Geometry: final body of the model. Coordinates: model frame, mm. Give positions to 0.01 mm unless a question says otherwise; leave off trailing zeros. Order: outer loops, then holes, each group sorted by start corner. A loop starts at its lowest first (then second) coordinate and runs counter-clockwise, first axis right, second up. Notation, with made-up numbers: (84, -22) - (139, -22) arc R31 ccw to (139, 17) - close; hole circle Ø6 at (58.25, 65). An arc over 180 degrees is marked (long way). One line per item, written item: value.
```python
from build123d import *

# Parameters (mm, degrees)
SKETCH1_W                   = 50.8
SKETCH1_H                   = 508
BOSS_EXTRUDE1_DEPTH         = 3.175
M2_5_CLEARANCE_HOLE1_D      = 2.9
F_1_4_0_25_DIAMETER_HOLE1_D = 6.35
SKETCH6_W                   = 3.175
SKETCH6_H                   = 19.05
BOSS_EXTRUDE2_DEPTH         = 4.7625
CRVPATTERN1_START           = 25.4
CRVPATTERN1_OUTLINE_W       = 19.05
CRVPATTERN1_OUTLINE_H       = 3.175
CRVPATTERN1_DEPTH           = 4.7625
F_10_CLEARANCE_HOLE1_D      = 5.1054


# Read off the part's stored shape, not the designer's step: CrvPattern1
with BuildPart() as part:
    # Sketch1 → Boss-Extrude1 (new body)
    with BuildSketch(Plane.XY):
        Rectangle(SKETCH1_W, SKETCH1_H)
    extrude(amount=BOSS_EXTRUDE1_DEPTH)

    # M2.5 Clearance Hole1 (through all)
    with Locations(Plane.XY.offset(3.175)):
        with Locations((-11, 244.65), (-7.778174593, 236.871825407), (0, 233.65), (7.778174593, 236.871825407), (11, 244.65)):
            Hole(M2_5_CLEARANCE_HOLE1_D / 2)

    # 1/4 (0.25) Diameter Hole1 (through all)
    with Locations(Plane.XY.offset(3.175)):
        with Locations((0, 244.65)):
            Hole(F_1_4_0_25_DIAMETER_HOLE1_D / 2)

    # Sketch6 → Boss-Extrude2 (add)
    with BuildSketch(Plane(origin=(25.4, 0, 0), x_dir=(0, 0, -1), z_dir=(1, 0, 0))):
        with Locations((-1.5875, -231.775)):
            Rectangle(SKETCH6_W, SKETCH6_H)
    boss_extrude2 = extrude(amount=BOSS_EXTRUDE2_DEPTH)

    # CrvPattern1 outline → CrvPattern1 (add)
    with BuildSketch(Plane.YZ.offset(CRVPATTERN1_START)):
        with Locations((-172.810714286, 1.5875)):
            Rectangle(CRVPATTERN1_OUTLINE_W, CRVPATTERN1_OUTLINE_H)
        with Locations((-113.846428571, 1.5875)):
            Rectangle(CRVPATTERN1_OUTLINE_W, CRVPATTERN1_OUTLINE_H)
        with Locations((-54.882142857, 1.5875)):
            Rectangle(CRVPATTERN1_OUTLINE_W, CRVPATTERN1_OUTLINE_H)
        with Locations((4.082142857, 1.5875)):
            Rectangle(CRVPATTERN1_OUTLINE_W, CRVPATTERN1_OUTLINE_H)
        with Locations((63.046428571, 1.5875)):
            Rectangle(CRVPATTERN1_OUTLINE_W, CRVPATTERN1_OUTLINE_H)
        with Locations((122.010714286, 1.5875)):
            Rectangle(CRVPATTERN1_OUTLINE_W, CRVPATTERN1_OUTLINE_H)
        with Locations((180.975, 1.5875)):
            Rectangle(CRVPATTERN1_OUTLINE_W, CRVPATTERN1_OUTLINE_H)
    crvpattern1 = extrude(amount=CRVPATTERN1_DEPTH)

    # Mirror1: Boss-Extrude2, CrvPattern1 across plane
    add(boss_extrude2.mirror(Plane.ZY))
    add(crvpattern1.mirror(Plane.ZY))

    # #10 Clearance Hole1 (through all)
    with Locations(Plane.XY.offset(3.175)):
        with Locations((16.002, -247.65), (-16.002, -247.65), (16.002, -222.25), (-16.002, -222.25)):
            Hole(F_10_CLEARANCE_HOLE1_D / 2)


solid = part.part
```
1) Section A-A, the plane y = -212. Return loops of the section in (x, z) (3 decimals).
Answers below:
outline: (-25.4, 0) - (25.4, 0) - (25.4, 3.175) - (-25.4, 3.175) - close
2) Material intervals for line 1 along X through (y, z) = (-247.65, 1.35); line 2 along X through (y, z) = (244.65, 2.3) (3 decimals); line 3 along Y through (x, z) = (0, 0.8) (3 decimals), sorted ascending.
Answers below:
line 1: -25.4 to -18.55, -13.45 to 13.45, 18.55 to 25.4
line 2: -25.4 to -12.45, -9.55 to -3.175, 3.175 to 9.55, 12.45 to 25.4
line 3: -254 to 232.2, 235.1 to 241.475, 247.825 to 254
3) Section B-B, the plane z = 2.1. Count the separate pieces of the cut face and the enclosed holes in it, then the cut area to 3 significant figures.
Answers below:
separate pieces: 1
enclosed holes: 10
area: 27,100 mm^2
4) First-contact query: pin 1 (1 mm diameter, centred on y = -147.5, z = 2, fed in from -X); pin 2 (1 mm diameter, centred on x = -27.5, z = 2, fed in from -Y). Flat tips, straight axial feed; report the tip coordinate or a pass-through.
Answers below:
pin 1: x = -25.4
pin 2: y = -241.3
